Geometry: see drawing. Coordinates: mm, zero at the bounding-box minimum. A direction names the side the tool comes from. Give positions to 0.01 mm unless a question says otherwise; leave off trailing zeros. Loops run counter-clockwise (first coordinate to the right, second up) from the corner with the lowest first, then second, coordinate; pieces in that order, holes last. Notation, with made-up numbers: M 42,-14.5 L 52,-14.5 A15 cw 52,-4.5 Z; hole C 46.5,39 d5. An arc over 180 degrees is marked long. Return JSON: item names as keys, results as strings. Group by question number.
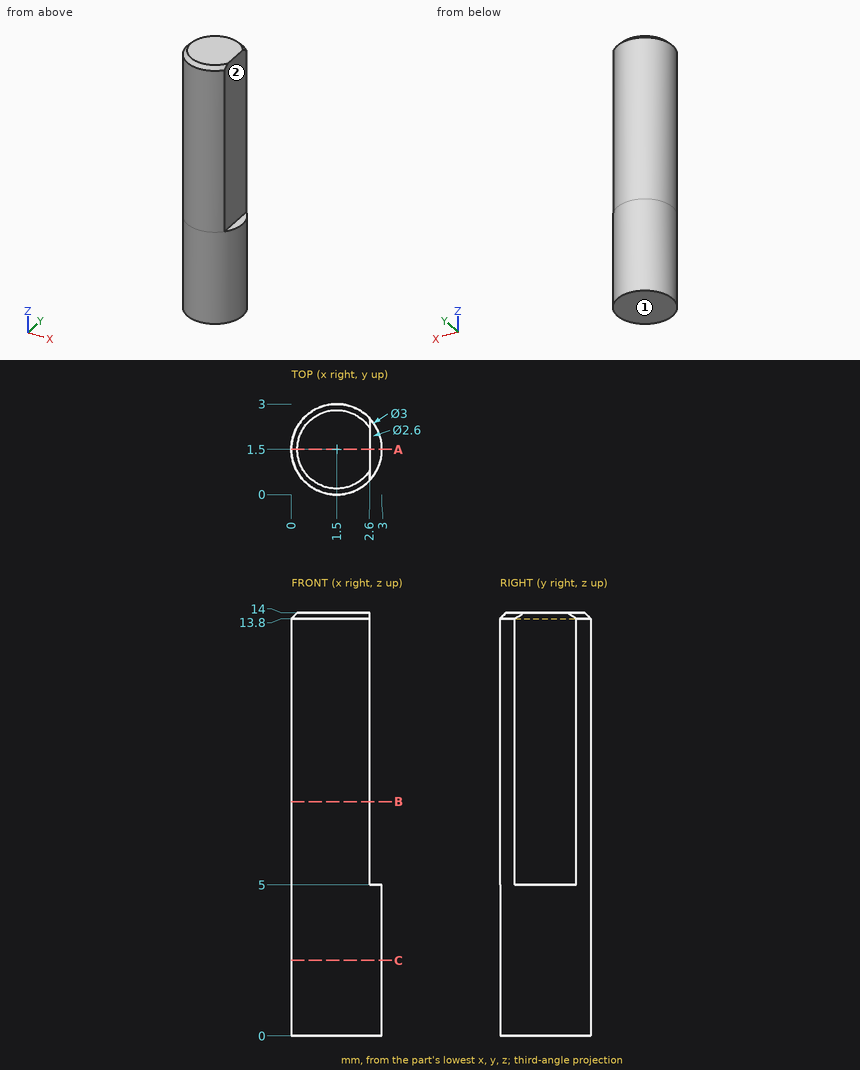
Item 1: Section B-B, the plane z = 7.75. Return loops of the section in (x, y).
Item 2: Section A-A, the plane y = 1.5. Return loops of the section in (x, z), then the cut area to 3 significant figures.
Item 3: Reachability of the marked faces 1 and 2 from +Z, -Z, +X, -X, +Y, -Y: full face, straight path, thin tool, end or side. Return the list, or none.
Item 4: Material intervals for line 1 (X direction, y = 0.75, z = 12); line 2 (Y direction, x = 0.4, z = 3); line 3 (X direction, y = 0.75, z = 3.25), sorted ascending. Write a range as from..to.
Item 5: First-contact query: pin 1 Ø1 at (y, z) = (2, 9.5) entering from +X. Flat tip, straight axial feed; report the tip coordinate or a pass-through.
Item 6: Section C-C, the plane z = 2.5. Return loops of the section in (x, y).
Answer below:
{
 "1": {"outline": "M 2.6,0.48 L 2.6,2.52 A1.5 ccw long Z"},
 "2": {"outline": "M 0,0 L 3,0 L 3,5 L 2.6,5 L 2.6,14 L 0.2,14 L 0,13.8 Z", "area": "38.4 mm^2"},
 "3": {"face 1": "-Z, +X, -X, +Y, -Y", "face 2": "+Z, +X, +Y, -Y"},
 "4": {"line 1": "0.2..2.6", "line 2": "0.48..2.52", "line 3": "0.2..2.8"},
 "5": {"pin 1": "x = 2.6"},
 "6": {"outline": "C 1.5,1.5 d3"}
}
